The model under review builds one solid part; all positions refer to its coordinate system, in mm. A direction names the side the tool comes from. Coordinates: 2 decimals unless noted, no trailing zeros. Loops run counter-clockwise (first coordinate to the right, second up) from the corner with the lowest first, then second, coordinate; pieces in that order, holes last. Notation, with made-up numbers: M -15.75,-30 L 7.25,-30 A15 ccw 7.25,-7 Z; hole C 25,2 d8. An arc over 180 degrees is marked long. One line per item, written item: value.
```python
from build123d import *

# Parameters (mm, degrees)
F0_W     = 118.5
F0_H     = 155.6
F0_R     = 9.5
F1_DEPTH = 4
F2_W     = 118.5
F2_H     = 155.6
F3_DEPTH = 5
F4_R     = 12.5
F4_W     = 118.5
F4_H     = 18.5
F5_DEPTH = 3


with BuildPart() as f1:
    # F0 (on Top) → F1 (new body)
    with BuildSketch(Plane.XY):
        Rectangle(F0_W, F0_H)
        with Locations((-35, -25)):
            Circle(F0_R, mode=Mode.SUBTRACT)
        with Locations((0, -25)):
            Circle(F0_R, mode=Mode.SUBTRACT)
        with Locations((35, -25)):
            Circle(F0_R, mode=Mode.SUBTRACT)
        with Locations((-35, 25)):
            Circle(F0_R, mode=Mode.SUBTRACT)
        with Locations((0, 25)):
            Circle(F0_R, mode=Mode.SUBTRACT)
        with Locations((35, 25)):
            Circle(F0_R, mode=Mode.SUBTRACT)
    extrude(amount=F1_DEPTH)

    # F2 (on face) → F3 (join)
    with BuildSketch(Plane.XY.offset(4)):
        Rectangle(F2_W, F2_H)
    extrude(amount=F3_DEPTH)

    # F4 (on face) → F5 (cut)
    with BuildSketch(Plane(origin=(0, 0, 0), x_dir=(1, 0, 0), z_dir=(0, 0, -1))):
        with Locations((-35, 25)):
            Circle(F4_R)
        with Locations((-35, -25)):
            Circle(F4_R)
        with Locations((0, 25)):
            Circle(F4_R)
        with Locations((0, -25)):
            Circle(F4_R)
        with Locations((35, 25)):
            Circle(F4_R)
        with Locations((35, -25)):
            Circle(F4_R)
        with Locations((0, 68.55)):
            Rectangle(F4_W, F4_H)
        with Locations((0, -68.55)):
            Rectangle(F4_W, F4_H)
    extrude(amount=-F5_DEPTH, mode=Mode.SUBTRACT)


solid = f1.part
```
(1) To check wall thickness, follow L1, parallel to Y at x = 0, z = 1.1; L2, parallel to X at y = 25, z = 3.45; L3, parallel to X at y = -25, z = 1.9. State the ranges of each line that lie inside material, in increasing order. Write a range as [from, to].
Checks:
L1: [-59.3, -37.5], [-12.5, 12.5], [37.5, 59.3]
L2: [-59.25, -44.5], [-25.5, -9.5], [9.5, 25.5], [44.5, 59.25]
L3: [-59.25, -47.5], [-22.5, -12.5], [12.5, 22.5], [47.5, 59.25]
(2) Add section A-A on x = 0. State the section outline as (y, z) points.
Checks:
outline: M -77.8,3 L -59.3,3 L -59.3,0 L -37.5,0 L -37.5,3 L -34.5,3 L -34.5,4 L -15.5,4 L -15.5,3 L -12.5,3 L -12.5,0 L 12.5,0 L 12.5,3 L 15.5,3 L 15.5,4 L 34.5,4 L 34.5,3 L 37.5,3 L 37.5,0 L 59.3,0 L 59.3,3 L 77.8,3 L 77.8,9 L -77.8,9 Z
(3) Tool access review of faces 4 (the face through (2.7, 15.7, 3)), 5 (the face through (-1, 1, 0)), 6 (the face through (-1, -69, 3)): name each direction out of +Z, -Z, +X, -X, +Y, -Y from which nothing blocks a thin tool from reaching the whole face with its end or side.
Checks:
face 4: -Z
face 5: -Z, +X, -X, +Y, -Y
face 6: -Z, +X, -X, -Y
(4) Add section C-C on x = -14.5. State the section outline as (y, z) points, then the cut area to 3 significant figures.
Checks:
outline: M -77.8,3 L -59.3,3 L -59.3,0 L 59.3,0 L 59.3,3 L 77.8,3 L 77.8,9 L -77.8,9 Z
area: 1,290 mm^2
(5) Add section D-D on y = 66.5. State the section outline as (x, z) points, then the cut area to 3 significant figures.
Checks:
outline: M -59.25,3 L 59.25,3 L 59.25,9 L -59.25,9 Z
area: 711 mm^2
(6) Insertion check: pin 1 Ø22 at (x, y) = (35, -25) entering from -Z; pin 2 Ø15 at (x, y) = (0, 25) entering from -Z. Each pin has a flat end and moves straight along its axis. Give the tip position at first contact, or say it passes through.
Checks:
pin 1: z = 3
pin 2: z = 4
(7) Add section B-B on y = 25. State the section outline as (x, z) points, then the cut area to 4 significant figures.
Checks:
outline: M -59.25,0 L -47.5,0 L -47.5,3 L -44.5,3 L -44.5,4 L -25.5,4 L -25.5,3 L -22.5,3 L -22.5,0 L -12.5,0 L -12.5,3 L -9.5,3 L -9.5,4 L 9.5,4 L 9.5,3 L 12.5,3 L 12.5,0 L 22.5,0 L 22.5,3 L 25.5,3 L 25.5,4 L 44.5,4 L 44.5,3 L 47.5,3 L 47.5,0 L 59.25,0 L 59.25,9 L -59.25,9 Z
area: 784.5 mm^2
(8) Draft analysis for pull direction X (two halves, no side actions). For faces 1 (the face through (-35, 25, 4)), 2 (the face through (-59.25, -1, 4)), 3 (the face through (-1, -77.8, 6)), state which applies: pulls with the +X half, pulls with the -X half, needs draft (parallel to the pull), parting line crosses it, or undercut.
Checks:
face 1: undercut
face 2: pulls with the -X half
face 3: needs draft
